from build123d import *

# Parameters (mm, degrees)
F1_DEPTH = 5


with BuildPart() as f1:
    # F0 (on Front) → F1 (new body)
    with BuildSketch(Plane.XZ):
        with BuildLine():
            Line((1.894506, -17.615913), (-27.500473, -34.587112))
            Line((-27.500473, -34.587112), (82.499527, -34.587112))
            Line((82.499527, -34.587112), (53.104548, -17.615913))
            ThreePointArc((53.104548, -17.615913), (51.606879, -14.899604), (53.313833, -12.309691))
            ThreePointArc((53.313833, -12.309691), (27.499527, 101.853226), (1.685221, -12.309691))
            ThreePointArc((1.685221, -12.309691), (3.392175, -14.899604), (1.894506, -17.615913))
        make_face()
    extrude(amount=F1_DEPTH)


solid = f1.part
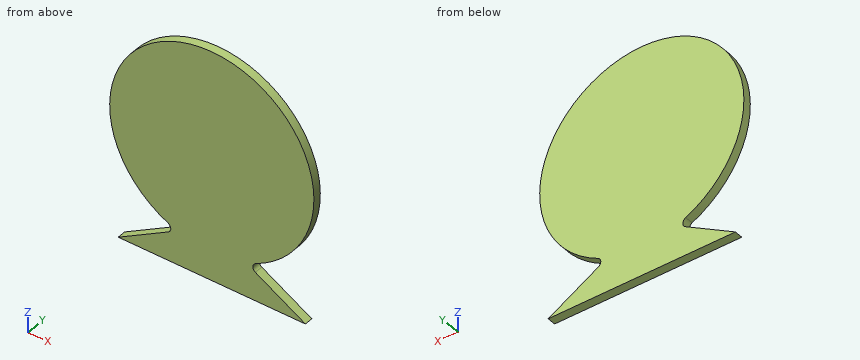
Geometry check sheet. Reference: the model listing, model coordinates, mm. Give positions to 0.01 mm unless a question says otherwise; leave off trailing zeros. Loops run counter-clockwise (first coordinate to the right, second up) from the corner with the lowest first, then second, coordinate; pieces in that order, holes last. Notation, with made-up numbers: M -25,48 L 22,48 A7 cw 22,56 Z; hole C 34.5,88 d1. An arc over 180 degrees is marked long. Write each question's results on one line, items separated by ' | '.
1) Thickness scan on line 1 (Z direction, x = 70.5, y = -2.25); line 2 (Z direction, x = 73.5, y = -4.25); line 3 (Z direction, x = 28, y = -4.4). Record the ranges inside material, lowest first.
Answers follow:
line 1: -34.59 to -27.66, 0.01 to 83.7 | line 2: -34.59 to -29.39, 3.33 to 80.38 | line 3: -34.59 to 101.85
2) Section check C-C, the plane x = -3. Record the boundary of the cut face in (y, z), plus the area to 3 significant figures.
Answers follow:
outline: M -5,-34.59 L 0,-34.59 L 0,-20.44 L -5,-20.44 Z; M -5,-9.82 L 0,-9.82 L 0,93.52 L -5,93.52 Z | area: 587 mm2
3) Gauge pin test, flat ends, axial feed: pin 1 (1 mm diameter, centred on y = -3.5, z = 68, fed in from -X); pin 2 (2 mm diameter, centred on y = -1, z = 84, fed in from +X); pin 3 (1 mm diameter, centred on x = 56.5, y = -4.5, fed in from +Z). Record the tip position at first contact, or that the pin passes through.
Answers follow:
pin 1: x = -26.74 | pin 2: x = 71.17 | pin 3: z = 94.65
4) Section check A-A, the plane x = 60. Record the boundary of the cut face in (y, z).
Answers follow:
outline: M -5,-34.59 L 0,-34.59 L 0,-21.6 L -5,-21.6 Z; M -5,-8.58 L 0,-8.58 L 0,92.29 L -5,92.29 Z
5) Section check B-B, the plane y = -1.95. Record the boundary of the cut face in (x, z).
Answers follow:
outline: M -27.5,-34.59 L 82.5,-34.59 L 53.1,-17.62 A3 cw 53.31,-12.31 A60 ccw long 1.69,-12.31 A3 cw 1.89,-17.62 Z
6) Section check D-D, the plane z = 73.5. Record the boundary of the cut face in (x, y), plus the area to 3 significant figures.
Answers follow:
outline: M -23.48,-5 L 78.47,-5 L 78.47,0 L -23.48,0 Z | area: 510 mm2
